Build history of the part. All positions in model axes, mm. A direction names the side the tool comes from. Round coordinates to 2 decimals unless told otherwise and drop trailing zeros. Order: outer loops, then holes, each group sorted by start corner. A loop starts at its lowest first (then second) coordinate and runs counter-clockwise, first axis right, second up. Notation, with made-up numbers: (69.5, 77.5) - (76.5, 77.5) arc R6 ccw to (76.5, 83.5) - close; hole circle Ø1 at (82.25, 22.25). An arc over 180 degrees is marked (long way). One line per question, with ' | ' between items. Start each with the question number.
from build123d import *

# Parameters (mm, degrees)
F0_W     = 66
F0_H     = 48
F0_R     = 1.1
F0_R_2   = 10
F1_DEPTH = 1.5
F2_R     = 2
F3_R     = 2.5
F4_DEPTH = 0.5


with BuildPart() as f1:
    # F0 (on Top) → F1 (new body)
    with BuildSketch(Plane.XY):
        Rectangle(F0_W, F0_H)
        with Locations((-25, -9.9985)):
            Circle(F0_R, mode=Mode.SUBTRACT)
        with Locations((0, -10.9985)):
            Circle(F0_R_2, mode=Mode.SUBTRACT)
        with Locations((25, -9.9985)):
            Circle(F0_R, mode=Mode.SUBTRACT)
        with Locations((-25, 9.9985)):
            Circle(F0_R, mode=Mode.SUBTRACT)
        with Locations((25, 9.9985)):
            Circle(F0_R, mode=Mode.SUBTRACT)
    extrude(amount=F1_DEPTH)

    # F2
    f2_edges = [f1.edges().sort_by_distance(p)[0] for p in [
        (-33, -24, 0.75),
        (33, -24, 0.75),
        (-33, 24, 0.75),
        (33, 24, 0.75),
    ]]
    fillet(f2_edges, radius=F2_R)

    # F3 (on face) → F4 (cut)
    with BuildSketch(Plane.XY.offset(1.5)):
        with Locations((-25, 9.9985)):
            Circle(F3_R)
        with Locations((25, 9.9985)):
            Circle(F3_R)
        with Locations((-25, -9.9985)):
            Circle(F3_R)
        with Locations((25, -9.9985)):
            Circle(F3_R)
    extrude(amount=-F4_DEPTH, mode=Mode.SUBTRACT)


solid = f1.part
Item 1: Pin check, flat tip, straight feed: pin 1 (1.5 mm diameter, centred on x = -24.5, y = 9.5, fed in from +Z). Stop position of the tip, or through.
Item 2: Slice it at B-B (x = 0). Write the cut outline in (y, z).
Item 3: Slice it at C-C (y = -20). Write the cut outline in (x, z).
Item 4: Pull direction Y, two halves, no side cores. Call faces 3 (the face through (-26.843, -8.309, 1.254)), 4 (the face through (0, 0, 1.5)), 5 (the face through (0, 24, 1)): released by +Y, released by -Y, zero draft, split by the parting line, or undercut.
Item 5: 3-axis set-ups, long thin cutter, end or side, ignore diameter. For faces 1 (the face through (-33, 0, 1)), 2 (the face through (23.16, 11.69, 1.25)): which of +Z, -Z, +X, -X, +Y, -Y reach the whole face in a straight line?
Item 6: Wall check: line 1 along Y through (x, z) = (25, 0.5); line 2 along Y through (x, z) = (-25, 1.15); line 3 along Y through (x, z) = (0, 0.5). Give the ranges that are in metal, low to high. Write a range as [from, to].
Item 7: Slice it at A-A (x = -25). Write the cut outline in (y, z), plus the area to 3 significant figures.
Item 8: Slice it at D-D (z = 0.75). Write the cut outline in (x, y), plus the area to 3 significant figures.
A:
1) pin 1: z = 1
2) outline: (-24, 0) - (-21, 0) - (-21, 1.5) - (-24, 1.5) - close; (-1, 0) - (24, 0) - (24, 1.5) - (-1, 1.5) - close
3) outline: (-33, 0) - (-4.36, 0) - (-4.36, 1.5) - (-33, 1.5) - close; (4.36, 0) - (33, 0) - (33, 1.5) - (4.36, 1.5) - close
4) face 3: undercut | face 4: zero draft | face 5: released by +Y
5) face 1: +Z, -Z, -X, +Y, -Y | face 2: +Z
6) line 1: [-24, -11.1], [-8.9, 8.9], [11.1, 24] | line 2: [-24, -12.5], [-7.5, 7.5], [12.5, 24] | line 3: [-24, -21], [-1, 24]
7) outline: (-24, 0) - (-11.1, 0) - (-11.1, 1) - (-12.5, 1) - (-12.5, 1.5) - (-24, 1.5) - close; (-8.9, 0) - (8.9, 0) - (8.9, 1) - (7.5, 1) - (7.5, 1.5) - (-7.5, 1.5) - (-7.5, 1) - (-8.9, 1) - close; (11.1, 0) - (24, 0) - (24, 1.5) - (12.5, 1.5) - (12.5, 1) - (11.1, 1) - close | area: 62.6 mm^2
8) outline: (-33, -22) arc R2 ccw to (-31, -24) - (31, -24) arc R2 ccw to (33, -22) - (33, 22) arc R2 ccw to (31, 24) - (-31, 24) arc R2 ccw to (-33, 22) - close; hole circle Ø2.2 at (-25, -10); hole circle Ø2.2 at (-25, 10); hole circle Ø20 at (0, -11); hole circle Ø2.2 at (25, -10); hole circle Ø2.2 at (25, 10) | area: 2,840 mm^2
